Geometry check sheet. Reference: the model listing, model coordinates, mm. Face numbers are marked on the shaded views. Round coordinates to 2 decimals unless told otherwise and drop trailing zeros. Loops run counter-clockwise (first coordinate to the right, second up) from the corner with the lowest first, then second, coordinate; pieces in that order, holes last. Notation, with made-up numbers: (-37.5, -18) -> (20.5, -18) arc R27 cw to (20.5, 9) -> close; hole circle Ø1 at (-19, 60). An arc over 180 degrees is marked (long way). Use a Markdown table: item, result. Add a question column.
Q1. Sectioned sample at B-B, the plane z = 10. Enter the section's corners in (x, y).
Q2. Material ranges on L1, parallel to X at y = 3.25, z = -10; L2, parallel to Z at x = -17, y = 0.75; L3, parallel to Y at x = -12, z = -0.25, recorded low to high.
Q3. Gauge pin test, flat ends, axial feed: P1, Ø2.5, axis at x = 10, z = -10, coming from the +Y side; P2, Ø3.5, axis at x = 2, z = 0.5, coming from the -Y side. Record the tip position at first contact, or that the pin passes through.
Q4. Sectioned sample at A-A, the plane y = 2.5. Enter the section's corners in (x, z).
Q5. Sectioned sample at C-C, the plane x = 10. Enter the section's corners in (y, z), then the cut area to 3 significant figures.
Q6. Release check for a two-part mould opening along Z. For the marked faces 1, 2, 3 and 4 record: released by +Z, released by -Z, zero draft, split by the parting line, or undercut.
Q7. Sectioned sample at D-D, the plane y = 4.5. Enter the section's corners in (x, z).
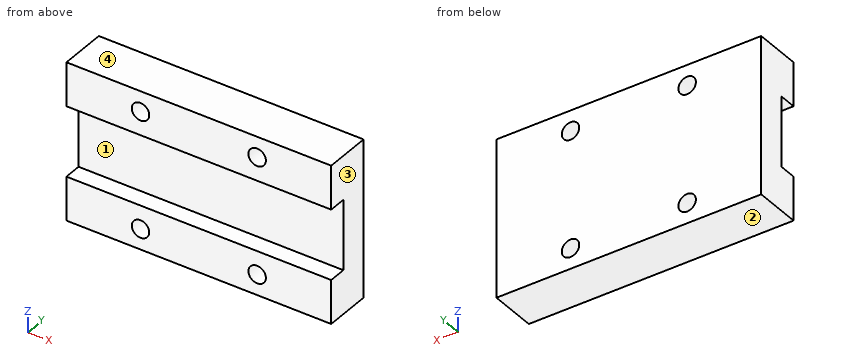
```python
from build123d import *

# Parameters (mm, degrees)
SKETCH1_W           = 45.4
SKETCH1_H           = 27
BOSS_EXTRUDE1_DEPTH = 8
SKETCH2_W           = 12
SKETCH2_H           = 3
CUT_EXTRUDE1_DEPTH  = 49.0355077
SKETCH3_R           = 1.5
CUT_EXTRUDE2_DEPTH  = 10


with BuildPart() as part:
    # Sketch1 → Boss-Extrude1 (new body)
    with BuildSketch(Plane(origin=(0, 0, 0), x_dir=(1, 0, 0), z_dir=(0, 1, 0))):
        Rectangle(SKETCH1_W, SKETCH1_H)
    extrude(amount=BOSS_EXTRUDE1_DEPTH)

    # Sketch2 → Cut-Extrude1 (cut, through all)
    with BuildSketch(Plane(origin=(22.7, 0, 0), x_dir=(0, 0, -1), z_dir=(1, 0, 0))):
        with Locations((0, 1.5)):
            Rectangle(SKETCH2_W, SKETCH2_H)
    extrude(amount=-CUT_EXTRUDE1_DEPTH, mode=Mode.SUBTRACT)

    # Sketch3 → Cut-Extrude2 (cut)
    with BuildSketch(Plane(origin=(0, 8, 0), x_dir=(1, 0, 0), z_dir=(0, 1, 0))):
        with Locations(Location((10, -10, 0), (0, 0, 270))):
            Circle(SKETCH3_R)
        with Locations(Location((-10, -10, 0), (0, 0, 270))):
            Circle(SKETCH3_R)
        with Locations(Location((-10, 10, 0), (0, 0, 270))):
            Circle(SKETCH3_R)
        with Locations(Location((10, 10, 0), (0, 0, 270))):
            Circle(SKETCH3_R)
    extrude(amount=-CUT_EXTRUDE2_DEPTH, mode=Mode.SUBTRACT)


solid = part.part
```
Values:
| question | item | result |
|---|---|---|
| 1 | outline | (-22.7, 0) -> (-11.5, 0) -> (-11.5, 8) -> (-22.7, 8) -> close; (-8.5, 0) -> (8.5, 0) -> (8.5, 8) -> (-8.5, 8) -> close; (11.5, 0) -> (22.7, 0) -> (22.7, 8) -> (11.5, 8) -> close |
| 2 | L1 | -22.7 to -11.5, -8.5 to 8.5, 11.5 to 22.7 |
| 2 | L2 | -13.5 to -6, 6 to 13.5 |
| 2 | L3 | 3 to 8 |
| 3 | P1 | through |
| 3 | P2 | y = 3 |
| 4 | outline | (-22.7, -13.5) -> (22.7, -13.5) -> (22.7, -6) -> (-22.7, -6) -> close; (-22.7, 6) -> (22.7, 6) -> (22.7, 13.5) -> (-22.7, 13.5) -> close; hole circle Ø3 at (-10, -10); hole circle Ø3 at (-10, 10); hole circle Ø3 at (10, -10); hole circle Ø3 at (10, 10) |
| 5 | outline | (0, -13.5) -> (8, -13.5) -> (8, -11.5) -> (0, -11.5) -> close; (0, -8.5) -> (8, -8.5) -> (8, 8.5) -> (0, 8.5) -> (0, 6) -> (3, 6) -> (3, -6) -> (0, -6) -> close; (0, 11.5) -> (8, 11.5) -> (8, 13.5) -> (0, 13.5) -> close |
| 5 | area | 132 mm^2 |
| 6 | face 1 | undercut |
| 6 | face 2 | released by -Z |
| 6 | face 3 | zero draft |
| 6 | face 4 | released by +Z |
| 7 | outline | (-22.7, -13.5) -> (22.7, -13.5) -> (22.7, 13.5) -> (-22.7, 13.5) -> close; hole circle Ø3 at (-10, -10); hole circle Ø3 at (-10, 10); hole circle Ø3 at (10, -10); hole circle Ø3 at (10, 10) |
